```python
from build123d import *

# Parameters (mm, degrees)
BOSS_EXTRUDE1_DEPTH = 12.7
FILLET1_R           = 2.54


with BuildPart() as part:
    # Sketch1 → Boss-Extrude1 (new body)
    with BuildSketch(Plane(origin=(0, 0, 0), x_dir=(1, 0, 0), z_dir=(0, 1, 0))):
        with BuildLine():
            ThreePointArc((-9.841918443, 8.026620793), (4.260142942, 11.964162408), (12.7, 0))
            ThreePointArc((12.7, 0), (12.349099919, -2.964748082), (11.315790364, -5.765664614))
            ThreePointArc((11.315790364, -5.765664614), (23.993952322, -3.244561181), (36.340951501, -7.071226105))
            ThreePointArc((36.340951501, -7.071226105), (36.414038972, 6.267321996), (49.751485572, 6.453669581))
            ThreePointArc((49.751485572, 6.453669581), (30.344153641, 36.906923092), (17.672267645, 70.722133981))
            ThreePointArc((17.672267645, 70.722133981), (8.792640174, 60.643133724), (-2.325024911, 68.181804248))
            ThreePointArc((-2.325024911, 68.181804248), (-1.446618844, 37.524798959), (-9.841918443, 8.026620793))
        make_face()
    extrude(amount=BOSS_EXTRUDE1_DEPTH)

    # Fillet1
    fillet1_edges = [part.edges().sort_by_distance(p)[0] for p in [
        (-9.841918443, 6.35, -8.026620793),
        (-2.325024911, 6.35, -68.181804248),
        (17.672267645, 6.35, -70.722133981),
        (49.751485572, 6.35, -6.453669581),
        (36.340951501, 6.35, 7.071226105),
        (11.315790364, 6.35, 5.765664614),
    ]]
    fillet(fillet1_edges, radius=FILLET1_R)


solid = part.part
```
Geometry check sheet. Reference: the model listing, model coordinates, mm. Round coordinates to 2 decimals unless told otherwise and drop trailing zeros. Order: outer loops, then holes, each group sorted by start corner. A loop starts at its lowest first (then second) coordinate and runs counter-clockwise, first axis right, second up. Notation, with made-up numbers: M 44,3 L 70,3 A29 cw 70,23 Z; hole C 59.25,79 d6. An arc over 180 degrees is marked long. Write item = value, one per line.
Q1. Scan lines: line 1 (X direction, y = 8.5, z = -49); line 2 (Z direction, x = 40, y = 5.5); line 3 (X direction, y = 9.5, z = -29). Record each from-to range of solid material in increasing order.
Answer block:
line_1 = -0.67 to 24.88
line_2 = -20.01 to -8.54
line_3 = -2.89 to 34.55
Q2. Section check B-B (x = 11). Enter the section's corners in (y, z).
Answer block:
outline = M 0,-61.18 L 12.7,-61.18 L 12.7,-6.35 L 0,-6.35 Z
Q3. Depth check by flat-ended pin: pin 1 Ø1.5 at (x, y) = (2, 9.5) entering from +Z; pin 2 Ø10 at (x, z) = (25.5, -8) entering from -Y; pin 3 Ø1.5 at (x, y) = (11, 5) entering from -Z. Enter the tip coordinate at first touch or a pass-through.
Answer block:
pin_1 = -12.4
pin_2 = 0
pin_3 = -61.49
Q4. Section check A-A (z = -39.5). Enter the section's corners in (x, y), plus the area to 3 significant figures.
Answer block:
outline = M -1.22,0 L 29.08,0 L 29.08,12.7 L -1.22,12.7 Z
area = 385 mm^2
Q5. Release check for a two-part mould opening along Z. For faces 1 (the flat face through (19, 0, -31)), 2 (the cylindrical face through (30.36, 6.261, -36.876)), 3 (the cylindrical face through (35.82, 6.26, -5.61)) record: released by +Z, released by -Z, zero draft, split by the parting line, or undercut.
Answer block:
face_1 = zero draft
face_2 = released by -Z
face_3 = undercut
